Solid Edge part; units mm, degrees
sketch "Sketch1" plane through (0, 0, 0) normal (0, 0, 1) x (1, 0, 0)
  line L0 (-33.7579, 34.8421) -> (-33.7579, -29.1579)
  line L1 (-33.7579, -29.1579) -> (30.2421, -29.1579)
  line L2 (30.2421, -29.1579) -> (30.2421, 34.8421)
  line L3 (30.2421, 34.8421) -> (-33.7579, 34.8421)
  line L4 (-41.7579, 42.8421) -> (-41.7579, -37.1579)
  line L5 (-41.7579, -37.1579) -> (38.2421, -37.1579)
  line L6 (38.2421, -37.1579) -> (38.2421, 42.8421)
  line L7 (38.2421, 42.8421) -> (-41.7579, 42.8421)
  dimension "D1" = 38.2421
  dimension "D2" = 38.2421
  dimension "D3" = 30.2421
extrude "Protrusion1" add sketch "Sketch1" along normal blind 400
hole "Hole_10" at (-31.7579, -37.1579, 335) direction (0, 1, 0) diameter 6.2 depth 10
hole "Hole1" at (-31.7579, -37.1579, 297.5) direction (0, 1, 0) diameter 6.2 depth 10
hole "Hole2" at (-31.7579, -37.1579, 237.5) direction (0, 1, 0) diameter 6.2 depth 10
hole "Hole3" at (-31.7579, -37.1579, 200) direction (0, 1, 0) diameter 6.2 depth 10
hole "Hole4" at (-31.7579, -37.1579, 162.5) direction (0, 1, 0) diameter 6.2 depth 10
hole "Hole5" at (-31.7579, -37.1579, 102.5) direction (0, 1, 0) diameter 6.2 depth 10
hole "Hole6" at (-31.7579, -37.1579, 65) direction (0, 1, 0) diameter 6.2 depth 10
hole "Hole7" at (-31.7579, -37.1579, 27.5) direction (0, 1, 0) diameter 6.2 depth 10
hole "Hole8" at (-31.7579, -37.1579, 372.5) direction (0, 1, 0) diameter 6.2 depth 10
hole "Hole_19" at (-21.7579, 42.8421, 15) direction (0, -1, 0) diameter 8.5 end up to next
hole "Hole9" at (-21.7579, 42.8421, 55) direction (0, -1, 0) diameter 8.5 end up to next
hole "Hole10" at (18.2421, 42.8421, 55) direction (0, -1, 0) diameter 8.5 end up to next
hole "Hole11" at (18.2421, 42.8421, 345) direction (0, -1, 0) diameter 8.5 end up to next
hole "Hole12" at (18.2421, 42.8421, 385) direction (0, -1, 0) diameter 8.5 end up to next
hole "Hole13" at (-21.7579, 42.8421, 385) direction (0, -1, 0) diameter 8.5 end up to next
hole "Hole14" at (-21.7579, 42.8421, 345) direction (0, -1, 0) diameter 8.5 end up to next
hole "Hole15" at (18.2421, 42.8421, 15) direction (0, -1, 0) diameter 8.5 end up to next
The model under review builds one solid part; all positions refer to its coordinate system, in mm. A direction names the side the tool comes from. Coordinates: 2 decimals unless noted, no trailing zeros. Write each loop counter-clockwise with the first axis right and the second up, starting at its lowest first coordinate (ties: lowest second). Pieces come first, ordered by that corner, then holes. Notation, with made-up numbers: (-9, 17) -> (45, 17) arc R21 cw to (45, 52) -> close; hole circle Ø8 at (27.25, 72.5). An arc over 180 degrees is marked (long way). One line per item, written item: value. Start each with the question number.
Q1. Clearance check with a flat-ended pin moving along its axis: P1, Ø3.5, axis at x = -31.76, z = 335, coming from the -Y side. State where the tip first meets the part, or that it passes through.
Q2. The part is to be moulded in two halves that separate along Y. For faces 1 (the face through (-1, 34.842, 197)), 2 (the face through (-1, 42.842, 197)), 3 (the face through (-21.571, 38.898, 340.754)), 4 (the face through (-33.758, 3, 197)), say which applies: +Y half, -Y half, draft (parallel to the pull), parting line (faces both ways), or undercut.
Q3. To check wall thickness, follow probe 1 along X at (y, z) = (39, 385); probe 2 along Y at (x, z) = (-6, 373); probe 3 along X at (y, z) = (30, 204). State the ranges of each line that lie inside material, in increasing order.
Q4. Add section C-C, the plane z = 266. Give the boundary of the cut face in (x, y), then the cut area to 3 significant figures.
Q5. Add section B-B, the plane x = 4.5. Give the boundary of the cut face in (y, z).
Q6. For faces 5 (the face through (14.093, 38.898, 14.079)), 6 (the face through (-2, -37.158, 197)), 7 (the face through (30.242, 2, 197)), list the 3-axis set-ups (+Z, -Z, +X, -X, +Y, -Y) from which the entire face can be reached by the end or side of a thin tool; tool diameter is ignored.
Q7. Add section A-A, the plane y = 19. Give the boundary of the cut face in (x, z), then the cut area to 3 significant figures.
Response:
1. P1: y = 34.84
2. face 1: undercut
2. face 2: +Y half
2. face 3: draft
2. face 4: undercut
3. probe 1: -41.76 to -26.01, -17.51 to 13.99, 22.49 to 38.24
3. probe 2: -37.16 to -29.16, 34.84 to 42.84
3. probe 3: -41.76 to -33.76, 30.24 to 38.24
4. outline: (-41.76, -37.16) -> (38.24, -37.16) -> (38.24, 42.84) -> (-41.76, 42.84) -> close; hole (-33.76, -29.16) -> (30.24, -29.16) -> (30.24, 34.84) -> (-33.76, 34.84) -> close
4. area: 2,300 mm²
5. outline: (-37.16, 0) -> (-29.16, 0) -> (-29.16, 400) -> (-37.16, 400) -> close; (34.84, 0) -> (42.84, 0) -> (42.84, 400) -> (34.84, 400) -> close
6. face 5: +Y
6. face 6: +Z, -Z, +X, -X, -Y
6. face 7: +Z, -Z
7. outline: (-41.76, 0) -> (-33.76, 0) -> (-33.76, 400) -> (-41.76, 400) -> close; (30.24, 0) -> (38.24, 0) -> (38.24, 400) -> (30.24, 400) -> close
7. area: 6,400 mm²
